The listing builds one solid part. Answer for the finished solid, in the listing's coordinates (mm). Round coordinates to 2 decimals unless told otherwise and drop trailing zeros. Loops run counter-clockwise (first coordinate to the right, second up) from the corner with the lowest first, then second, coordinate; pieces in that order, holes last. Notation, with made-up numbers: (49, 80) - (96, 80) arc R30 cw to (96, 103) - close; hole circle Ø11 at (-9.75, 86). An arc over 180 degrees is marked (long way). One line per item, written item: value.
```python
from build123d import *

# Parameters (mm, degrees)
BOSS_EXTRUDE1_DEPTH = 3.175
CUT_EXTRUDE1_REACH  = 48.818
SKETCH2_R           = 11
CUT_EXTRUDE2_REACH  = 48.818
SKETCH3_W           = 25.4
SKETCH3_H           = 5.715
CUT_EXTRUDE4_REACH  = 48.818
SKETCH6_R           = 1.3250037
CUT_EXTRUDE6_DEPTH  = 47.817591721
SKETCH7_R           = 10
CUT_EXTRUDE7_DEPTH  = 47.817591721
FILLET1_R           = 6.35


with BuildPart() as part:
    # Sketch1 → Boss-Extrude1 (new body)
    with BuildSketch(Plane.XY):
        with BuildLine():
            Line((25.4, -13.800079969), (-25.4, -13.800079969))
            Line((-25.4, -13.800079969), (-25.4, 13.800079969))
            ThreePointArc((-25.4, 13.800079969), (0, 39.200079969), (25.4, 13.800079969))
            Line((25.4, 13.800079969), (25.4, -13.800079969))
        make_face()
    extrude(amount=BOSS_EXTRUDE1_DEPTH)

    # Sketch2 → Cut-Extrude1 (cut, up to next)
    with BuildSketch(Plane.XY.offset(3.175), mode=Mode.PRIVATE) as cut_extrude1_sk1:
        with Locations((0, 16.964919969)):
            Circle(SKETCH2_R)
    cut_extrude1_tool1 = extrude(cut_extrude1_sk1.sketch, amount=-CUT_EXTRUDE1_REACH, mode=Mode.PRIVATE) & part.part
    add(cut_extrude1_tool1.solids().sort_by_distance((0, 16.96492, 3.175))[0], mode=Mode.SUBTRACT)

    # Sketch3 → Cut-Extrude2 (cut, up to next)
    with BuildSketch(Plane.XY.offset(3.175), mode=Mode.PRIVATE) as cut_extrude2_sk1:
        with Locations((0, -10.942579969)):
            Rectangle(SKETCH3_W, SKETCH3_H)
    cut_extrude2_tool1 = extrude(cut_extrude2_sk1.sketch, amount=-CUT_EXTRUDE2_REACH, mode=Mode.PRIVATE) & part.part
    add(cut_extrude2_tool1.solids().sort_by_distance((0, -10.94258, 3.175))[0], mode=Mode.SUBTRACT)

    # Sketch5 → Cut-Extrude4 (cut, up to next)
    with BuildSketch(Plane.XY.offset(3.175), mode=Mode.PRIVATE) as cut_extrude4_sk1:
        Polygon((3.175, -4.275079969), (1.143, -4.275079969), (1.143, -8.085079969), (-1.143, -8.085079969), (-1.143, -4.275079969), (-3.175, -4.275079969), (-3.175, -1.735079969), (-1.143, -1.735079969), (-1.143, 7.154920031), (1.143, 7.154920031), (1.143, -1.735079969), (3.175, -1.735079969), align=None)
    cut_extrude4_tool1 = extrude(cut_extrude4_sk1.sketch, amount=-CUT_EXTRUDE4_REACH, mode=Mode.PRIVATE) & part.part
    add(cut_extrude4_tool1.solids().sort_by_distance((0, -1.045651, 3.175))[0], mode=Mode.SUBTRACT)

    # Sketch6 → Cut-Extrude6 (cut, through all)
    with BuildSketch(Plane.XY):
        with Locations((0, 30.464919969)):
            Circle(SKETCH6_R)
        with Locations((11.691342951, 10.214919969)):
            Circle(SKETCH6_R)
        with Locations((-11.691342951, 10.214919969)):
            Circle(SKETCH6_R)
    extrude(amount=CUT_EXTRUDE6_DEPTH, mode=Mode.SUBTRACT)

    # Sketch7 → Cut-Extrude7 (cut, through all)
    with BuildSketch(Plane.XY):
        with Locations((0, 10.964920031)):
            Circle(SKETCH7_R)
    extrude(amount=CUT_EXTRUDE7_DEPTH, mode=Mode.SUBTRACT)

    # Fillet1
    fillet1_edges = [part.edges().sort_by_distance(p)[0] for p in [
        (9.921567423, 12.214919982, 1.5875),
        (-9.921567423, 12.214919982, 1.5875),
    ]]
    fillet(fillet1_edges, radius=FILLET1_R)


solid = part.part
```
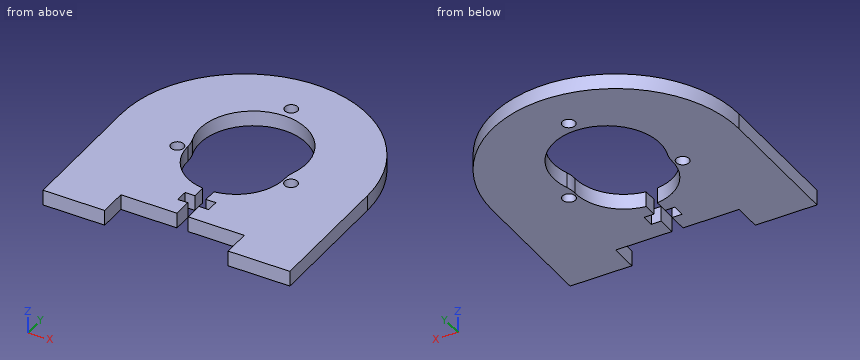
1) A cutting plane is placed at B-B on y = 20. Give the vertices of the cut face in (x, z) (3 decimals), and give its area (3 significant figures).
Final values:
outline: (-24.632, 0) - (-10.573, 0) - (-10.573, 3.175) - (-24.632, 3.175) - close; (10.573, 0) - (24.632, 0) - (24.632, 3.175) - (10.573, 3.175) - close
area: 89.3 mm2
2) A cutting plane is placed at C-C on z = 1.7. Give the number of separate pieces and of enclosed holes in the cut face, and give its area (3 significant figures).
Final values:
separate pieces: 1
enclosed holes: 3
area: 1,750 mm2
3) A cutting plane is placed at A-A on x = 0. Give the vertices of the cut face in (y, z) (3 decimals), and give its area (3 significant figures).
Final values:
outline: (27.965, 0) - (29.14, 0) - (29.14, 3.175) - (27.965, 3.175) - close; (31.79, 0) - (39.2, 0) - (39.2, 3.175) - (31.79, 3.175) - close
area: 27.3 mm2
4) Consider L1, parallel to X at y = -1.5, z = 1.1; L2, parallel to X at y = -3.5, z = 2.8 (3 decimals); L3, parallel to Y at x = 0, z = 1.15. Determine where each line is inside the solid, lowest interval first.
Final values:
L1: -25.4 to -1.14, 1.14 to 25.4
L2: -25.4 to -3.175, 3.175 to 25.4
L3: 27.96 to 29.14, 31.79 to 39.2
5) A cutting plane is placed at D-D on x = -17.5. Give the vertices of the cut face in (y, z) (3 decimals).
Final values:
outline: (-13.8, 0) - (32.21, 0) - (32.21, 3.175) - (-13.8, 3.175) - close
6) Each of these flat-tipped pins is pushed along its axis until it touches: pin 1 Ø1 at (x, z) = (-8.5, 1) entering from -Y; pin 2 Ø1 at (x, z) = (-2, 2) entering from +Y; pin 3 Ø1.5 at (x, z) = (-12.5, 1) entering from +Y. Where does it stop, or does it pass through?
Final values:
pin 1: y = -8.09
pin 2: y = 39.16
pin 3: y = 36.32
